Work out the finished part from the listing and answer in its coordinate system (mm). A direction names the side the tool comes from. Coordinates: 2 decimals unless noted, no trailing zeros. Order: outer loops, then holes, each group sorted by start corner. A loop starts at its lowest first (then second) coordinate and runs counter-clockwise, first axis right, second up. Notation, with made-up numbers: M 88.25,40.5 L 94.25,40.5 A34 cw 94.25,70.5 Z; hole C 73,-18.5 d5. An arc over 180 degrees is marked long. Write item = value, one per line. Start each with the question number.
Q1. Find section D-D on y = -118. Give the vertices of the cut face in (x, z).
Q2. Each of these flat-tipped pins is pushed along its axis until it touches: P1, Ø16, axis at y = -114, z = 1.5, coming from the +X side; P2, Ø12, axis at y = -69, z = -2.5, coming from the -X side; P3, Ø3, axis at x = 19.5, z = -2, coming from the -Y side. Where does it stop, or does it pass through?
Q3. Straight lines are drawn through the part: line 1 along Z through (x, y) = (18.5, -141); line 2 along Z through (x, y) = (-8, -16); line 3 along Y through (x, z) = (10, -3). For each, find the intervals that lie inside material, in ascending order.
Q4. Find section C-C on z = 0. Give the vertices of the cut face in (x, y), and give its area (3 significant figures).
Q5. A tool of negligible diameter and unlimited length cuts with its end or side. For faces 5 (the flat face through (-20, -30, 0)), 6 (the flat face through (0, 0, 0)), 7 (the flat face through (20, -30, 0)), from which of +Z, -Z, +X, -X, +Y, -Y can it reach the whole face along a straight path? Write none if from no direction.
Q6. Determine the mould class of faces 1 (the flat face through (-15, -91, 0)), 2 (the flat face through (0, -74, 20)), 3 (the flat face through (20, -91, -10)), 4 (the flat face through (0, -150, 0)) for opening direction Z: released by +Z, released by -Z, zero draft, split by the parting line, or undercut.
Q7. Find section B-B on x = -19.5. Give the vertices of the cut face in (y, z).
Q8. Find section A-A on y = -16. Give the vertices of the cut face in (x, z).
```python
from build123d import *

# Parameters (mm, degrees)
F0_W     = 50
F0_H     = 40
F1_DEPTH = 150
F2_R     = 5
F3_DEPTH = 104
F5_W     = 15
F5_H     = 20
F6_DEPTH = 120


with BuildPart() as f1:
    # F0 (on Front) → F1 (new body)
    with BuildSketch(Plane.XZ):
        Rectangle(F0_W, F0_H)
    extrude(amount=F1_DEPTH)


with BuildPart() as f3:
    # F2 (on face) → F3 (new body)
    with BuildSketch(Plane.YZ.offset(25)):
        with Locations((-16, 0)):
            Circle(F2_R)
    extrude(amount=-F3_DEPTH)


with BuildPart() as f1_1:
    add(f1.part)

    # F4: cut F3
    add(f3.part, mode=Mode.SUBTRACT)


with BuildPart() as f6:
    # F5 (on face) → F6 (new body)
    with BuildSketch(Plane.XZ.offset(150)):
        with Locations((-22.5, 0)):
            Rectangle(F5_W, F5_H)
        with Locations((22.5, 0)):
            Rectangle(F5_W, F5_H)
    extrude(amount=-F6_DEPTH)


with BuildPart() as f1_2:
    add(f1_1.part)

    # F7: cut F6
    add(f6.part, mode=Mode.SUBTRACT)


solid = f1_2.part
```
Findings below:
q1.outline = M -25,-20 L 25,-20 L 25,-10 L 15,-10 L 15,10 L 25,10 L 25,20 L -25,20 L -25,10 L -15,10 L -15,-10 L -25,-10 Z
q2.P1 = 15
q2.P2 = -15
q2.P3 = -30
q3.line_1 = -20 to -10, 10 to 20
q3.line_2 = -20 to -5, 5 to 20
q3.line_3 = -150 to -20, -12 to 0
q4.outline = M -25,-30 L -15,-30 L -15,-150 L 15,-150 L 15,-30 L 25,-30 L 25,-21 L -25,-21 Z; M -25,-11 L 25,-11 L 25,0 L -25,0 Z
q4.area = 4,600 mm^2
q5.face_5 = -X, -Y
q5.face_6 = +Z, -Z, +X, -X, +Y
q5.face_7 = +X, -Y
q6.face_1 = undercut
q6.face_2 = released by +Z
q6.face_3 = undercut
q6.face_4 = zero draft
q7.outline = M -150,-20 L 0,-20 L 0,20 L -150,20 L -150,10 L -30,10 L -30,-10 L -150,-10 Z; hole C -16,0 d10
q8.outline = M -25,-20 L 25,-20 L 25,-5 L -25,-5 Z; M -25,5 L 25,5 L 25,20 L -25,20 Z
